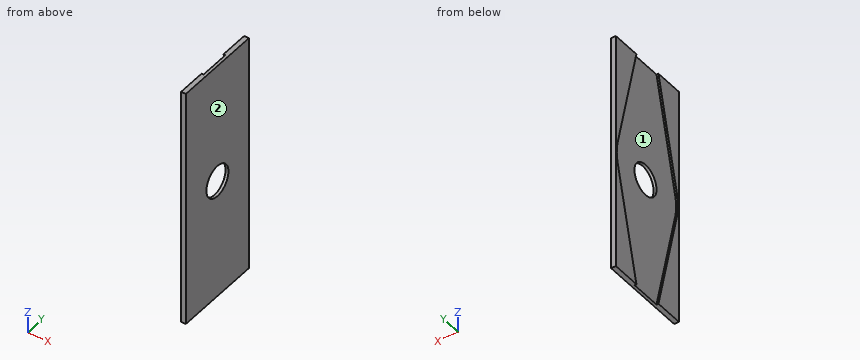
Autodesk Inventor part; units mm, degrees
ref_plane "YZ Plane" through (0, 0, 0) normal (1, 0, 0) x (0, 1, 0)
ref_plane "XZ Plane" through (0, 0, 0) normal (0, 1, 0) x (-1, 0, 0)
ref_plane "XY Plane" through (0, 0, 0) normal (0, 0, 1) x (1, 0, 0)
sketch "Sketch1" plane through (0, 0, 0) normal (0, 1, 0) x (-1, 0, 0)
  line L0 (95, 271.4286) -> (85, 271.4286)
  line L1 (85, 271.4286) -> (85, -224.5714)
  line L2 (85, -224.5714) -> (95, -224.5714)
  line L3 (95, -224.5714) -> (95, 271.4286)
  point P0 (0, 0)
  dimension "d0" = 10
  dimension "d1" = 496
extrude "Extrusion1" add sketch "Sketch1" along normal blind 186
sketch "Sketch3" plane through (-85, 0, 271.4286) normal (1, 0, 0) x (0, 0, -1)
  line L0 (0, 0) -> (496, 0)
  line L1 (496, 0) -> (496, 186)
  line L2 (0, 186) -> (496, 186)
  line L3 (0, 0) -> (0, 186)
  circle A0 centre (0, 93) radius 5
  line L4 (0, 0) -> (496, 0)
  circle A1 centre (248, 0) radius 5
  line L5 (0, 0) -> (248, 0)
  line L6 (0, 93) -> (0, 0)
  circle A2 centre (248, 93) radius 32.5
  point P0 (271.4286, 0)
  dimension "d16" = 65
  dimension "d19" = 93
  dimension "d20" = 248
  dimension "d21" = 248
  dimension "d22" = 93
extrude "Extrusion5" cut sketch "Sketch3" against normal blind 186 contours A2
sketch "Sketch5" plane through (-95, 0, -224.5714) normal (-1, 0, 0) x (0, 0, 1)
  circle A0 centre (248, 93) radius 32.5
  circle A1 centre (248, 93) radius 90.5
  line L0 (0, 0) -> (0, 186)
  circle A2 centre (0, 93) radius 32.5
  line L1 (496, 0) -> (496, 186)
  circle A3 centre (496, 93) radius 32.5
  line L2 (0, 60.5) -> (226.495, 5.0922)
  line L3 (0, 125.5) -> (224.5714, 180.4148)
  line L4 (496, 125.5) -> (269.505, 180.9078)
  line L5 (496, 60.5) -> (271.4286, 5.5852)
  point P0 (224.5714, 0)
  dimension "d23" = 181
extrude "Extrusion6" cut sketch "Sketch5" against normal blind 4 contours A1 | A1 L4 A3 L5 | A1 L2 A2 L3 | L1 A3 | A2 L0 picked at (485.2457, 91.6942) picked at (6.7545, 84.5302)
properties part number "Osnova" material "Aluminum 6061"
Here's how the part is built. I have some questions about the finished solid (model axes, mm). Face numbers are marked on the shaded views. Give positions to 0.01 mm unless a question says otherwise; leave off trailing zeros. Loops run counter-clockwise (first coordinate to the right, second up) from the corner with the lowest first, then second, coordinate; pieces in that order, holes last. Notation, with made-up numbers: (23.5, -1) -> (47.5, -1) arc R27 ccw to (47.5, 28) -> close; hole circle Ø3 at (-23, 26). An arc over 180 degrees is marked (long way). Answer as a JSON object with one key per item and string values. Group by question number.
Item 1: I need wall thicknesses on L1, parallel to Y at x = -91.5, z = -180; L2, parallel to X at y = 98, z = 222; L3, parallel to Y at x = -94.5, z = 6.5. Which ranges of each line are inside material? Lowest first, please.
Item 2: Will this pin go through, and if not, where does the flat tip stop? pin 1 (2 mm diameter, centred on y = 157, z = -87.5, fed in from -X).
Item 3: Imagine slicing it at A-A on y = 93. Write out the boundary of the cut face in (x, z), then the cut area to 3 significant figures.
Item 4: Thinking about a two-plate mould opening in Y: for the marked faces 1 and 2, which applies, pulls with the +Y half, pulls with the -Y half, needs draft (parallel to the pull), parting line crosses it, or undercut?
Item 5: Imagine slicing it at B-B on x = -88. Write out the boundary of the cut face in (y, z).
Item 6: Imagine slicing it at C-C on z = 39.5. Write out the boundary of the cut face in (x, y).
Item 7: Imagine slicing it at D-D on y = 29.5. Write out the boundary of the cut face in (x, z), then the cut area to 3 significant figures.
Answer list:
{
 "1": {"L1": "y = 0 to 49.6, 136.4 to 186", "L2": "x = -91 to -85", "L3": "y = 0 to 4.1, 181.9 to 186"},
 "2": {"pin 1": "stops at x = -91"},
 "3": {"outline": "(-91, -224.57) -> (-85, -224.57) -> (-85, -9.07) -> (-91, -9.07) -> close; (-91, 55.93) -> (-85, 55.93) -> (-85, 271.43) -> (-91, 271.43) -> close", "area": "2,590 mm2"},
 "4": {"face 1": "undercut", "face 2": "needs draft"},
 "5": {"outline": "(0, -224.57) -> (186, -224.57) -> (186, 271.43) -> (0, 271.43) -> close; hole circle Ø65 at (93, 23.43)"},
 "6": {"outline": "(-95, 0) -> (-85, 0) -> (-85, 64.75) -> (-91, 64.75) -> (-91, 3.94) -> (-95, 3.94) -> close; (-95, 182.06) -> (-91, 182.06) -> (-91, 121.25) -> (-85, 121.25) -> (-85, 186) -> (-95, 186) -> close"},
 "7": {"outline": "(-95, -224.57) -> (-85, -224.57) -> (-85, 271.43) -> (-95, 271.43) -> (-95, 144.66) -> (-91, 144.66) -> (-91, -97.85) -> (-95, -97.85) -> close", "area": "3,990 mm2"}
}
